from build123d import *
from OCP.BRepAlgoAPI import BRepAlgoAPI_Cut
from OCP.TopTools import TopTools_ListOfShape
from build123d.topology import SkipClean

# Parameters (mm, degrees)
SKETCH1_R                   = 6
EXTRUDE1_DEPTH              = 10
SKETCH2_R                   = 10.75
CUT_EXTRUDE1_DEPTH          = 6
SKETCH3_R                   = 1.6
CUT_EXTRUDE2_DEPTH          = 8.999999347
SKETCH4_W                   = 7
SKETCH4_H                   = 10
SKETCH4_R                   = 1.6
EXTRUDE3_DEPTH              = 9
FILLET2_R                   = 5
CHAMFER4_SIZE               = 6
CHAMFER4_SIZE2              = 10.392304845
M4_TAPPED_HOLE1_D           = 3.3
M4_TAPPED_HOLE1_DEPTH       = 10.1
M4_TAPPED_HOLE1_TIP         = 0.991420021
SKETCH6_R                   = 1.25
EXTRUDE4_DEPTH              = 4
M3_START                    = 12.4999999
M3_TAPPED_HOLE1_OUTLINE_R   = 1.25
M3_TAPPED_HOLE1_DEPTH       = 0.5000001
M3_START_2                  = -13
M3_TAPPED_HOLE1_2_OUTLINE_R = 1.25
M3_TAPPED_HOLE1_2_DEPTH     = 0.4999999
EXTRUDE5_REACH              = 36.756
SKETCH8_W                   = 6
SKETCH8_H                   = 4.052940251


with BuildPart() as part:
    # Sketch1 → Extrude1 (new body)
    with BuildSketch(Plane.XY):
        Polygon((-17, 6.53e-07), (-28, 6.53e-07), (-28, -8.999999347), (28, -8.999999347), (28, 0), (17, 0), (17, 18.000000653), (-17, 18.000000653), align=None)
        with Locations((0, 6.53e-07)):
            Circle(SKETCH1_R, mode=Mode.SUBTRACT)
    extrude(amount=EXTRUDE1_DEPTH)

    # Sketch2 → Cut-Extrude1 (cut)
    with BuildSketch(Plane(origin=(0, 0, 0), x_dir=(-1, 0, 0), z_dir=(0, 0, -1))):
        Circle(SKETCH2_R)
    extrude(amount=-CUT_EXTRUDE1_DEPTH, mode=Mode.SUBTRACT)


with BuildPart() as cut_extrude2_tool:
    # Sketch3 → Cut-Extrude2 (new body)
    with BuildSketch(Plane(origin=(0, 0, 0), x_dir=(-1, 0, 0), z_dir=(0, 1, 0))):
        with Locations(Location((-24.5, 5, 0), (0, 0, 90))):
            Circle(SKETCH3_R)
        with Locations(Location((24.5, 5, 0), (0, 0, 90))):
            Circle(SKETCH3_R)
    extrude(amount=-CUT_EXTRUDE2_DEPTH)


with BuildPart() as part_1:
    add(part.part)

    # Cut-Extrude2: cut by cut_extrude2_tool, with a tolerance
    cut_extrude2_stock = TopTools_ListOfShape()
    cut_extrude2_stock.Append(part_1.part.wrapped)
    cut_extrude2_tools = TopTools_ListOfShape()
    cut_extrude2_tools.Append(cut_extrude2_tool.part.wrapped)
    cut_extrude2_cut = BRepAlgoAPI_Cut()
    cut_extrude2_cut.SetArguments(cut_extrude2_stock)
    cut_extrude2_cut.SetTools(cut_extrude2_tools)
    cut_extrude2_cut.SetFuzzyValue(0.00001)
    cut_extrude2_cut.Build()
    add(Compound.cast(cut_extrude2_cut.Shape()).solids(), mode=Mode.REPLACE)

    # Sketch4 → Extrude3 (add)
    # profile 1 of 2: a face of its own
    with SkipClean():  # the faces are left unmerged after this step: merging them gives an invalid solid
        with BuildSketch(Plane.XZ.offset(8.999999347)):
            with Locations((-24.5, 5)):
                Rectangle(SKETCH4_W, SKETCH4_H)
            with Locations((-24.5, 5)):
                Circle(SKETCH4_R, mode=Mode.SUBTRACT)
        # profile 2 of 2: a face of its own
        with BuildSketch(Plane.XZ.offset(8.999999347)):
            with Locations((24.5, 5)):
                Rectangle(SKETCH4_W, SKETCH4_H)
            with Locations((24.5, 5)):
                Circle(SKETCH4_R, mode=Mode.SUBTRACT)
        extrude(amount=EXTRUDE3_DEPTH)
    add(part_1.part.scale(1), mode=Mode.REPLACE)  # the faces are merged on a copy

    # Fillet2
    fillet2_edges = [part_1.edges().sort_by_distance(p)[0] for p in [
        (28, -13.499999347, 0),
        (28, -13.499999347, 10),
        (-28, -8.999999347, 0),
        (-28, -8.999999347, 10),
    ]]
    fillet(fillet2_edges, radius=FILLET2_R - 0.0001)  # a hair under: the kernel refuses the full size

    # Chamfer4
    chamfer4_edges = [part_1.edges().sort_by_distance(p)[0] for p in [
        (0, 18.000000653, 10),
    ]]
    chamfer4_side = [part_1.faces().sort_by_distance(p)[0] for p in [
        (0, 18.000000653, 5),
    ]]
    chamfer(chamfer4_edges, length=CHAMFER4_SIZE, length2=CHAMFER4_SIZE2, reference=chamfer4_side[0])

    # M4 Tapped Hole1
    with Locations(Plane(origin=(-24.5, -17.999999347, 5), x_dir=(0, 0, -1), z_dir=(0, -1, 0))):
        with Locations((0, 0), (0, 49)):
            Hole(M4_TAPPED_HOLE1_D / 2, depth=M4_TAPPED_HOLE1_DEPTH)
            with Locations((0, 0, -(M4_TAPPED_HOLE1_DEPTH + M4_TAPPED_HOLE1_TIP / 2))):  # 118° drill point
                Cone(0, M4_TAPPED_HOLE1_D / 2, M4_TAPPED_HOLE1_TIP, mode=Mode.SUBTRACT)

    # Sketch6 → Extrude4 (cut)
    with BuildSketch(Plane.ZY.offset(17)):
        with Locations((3.33604719, 14.150000653)):
            Circle(SKETCH6_R)
        with Locations((6.332495088, 8.960000653)):
            Circle(SKETCH6_R)
    extrude4 = extrude(amount=-EXTRUDE4_DEPTH, mode=Mode.SUBTRACT)

    # Mirror1: Extrude4 across plane
    add(extrude4.mirror(Plane(origin=(0, 0, 0), x_dir=(0, 0, 1), z_dir=(1, 0, 0))), mode=Mode.SUBTRACT)

    # M3 Tapped Hole1: read off the stored shape, not the designer's step
    # M3 Tapped Hole1 outline → M3 Tapped Hole1 (cut)
    with SkipClean():  # the faces are left unmerged after this step: merging them gives an invalid solid
        with BuildSketch(Plane.YZ.offset(M3_START)):
            with Locations((14.150000653, 3.33604719)):
                Circle(M3_TAPPED_HOLE1_OUTLINE_R)
            with Locations((8.960000653, 6.332495088)):
                Circle(M3_TAPPED_HOLE1_OUTLINE_R)
        extrude(amount=M3_TAPPED_HOLE1_DEPTH, mode=Mode.SUBTRACT)

    # M3 Tapped Hole1 2 outline → M3 Tapped Hole1 2 (cut)
    with BuildSketch(Plane.YZ.offset(M3_START_2)):
        with Locations((14.150000653, 3.33604719)):
            Circle(M3_TAPPED_HOLE1_2_OUTLINE_R)
        with Locations((8.960000653, 6.332495088)):
            Circle(M3_TAPPED_HOLE1_2_OUTLINE_R)
    extrude(amount=M3_TAPPED_HOLE1_2_DEPTH, mode=Mode.SUBTRACT)

    # M3 Tapped Hole1 3 outline → M3 Tapped Hole1 3 (revolve, cut)
    with BuildSketch(Plane(origin=(0, 14.150000653, 3.33604719), x_dir=(0, 1, 0), z_dir=(0, 0, -1))):
        Polygon((0, 12.5), (0, 11.748924226), (1.25, 12.5), align=None)
        Polygon((1.25, -12.5), (0, -11.748924226), (0, -12.5000001), align=None)
    revolve(axis=Axis((0, 14.150000653, 3.33604719), (1, 0, 0)), mode=Mode.SUBTRACT)

    # M3 Tapped Hole1 4 outline → M3 Tapped Hole1 4 (revolve, cut)
    with BuildSketch(Plane(origin=(0, 8.960000653, 6.332495088), x_dir=(0, 1, 0), z_dir=(0, 0, -1))):
        Polygon((0, 12.5), (0, 11.748924226), (1.25, 12.5), align=None)
        Polygon((1.25, -12.5), (0, -11.748924226), (0, -12.5000001), align=None)
    revolve(axis=Axis((0, 8.960000653, 6.332495088), (1, 0, 0)), mode=Mode.SUBTRACT)

    # Extrude5: up to this plane
    extrude5_end = Plane(origin=(-17, 7.607695808, 10), z_dir=(0, -0.5000000000000007, -0.8660254037844384))
    # Sketch8 → Extrude5 (cut, up to the surface)
    with BuildSketch(Plane(origin=(0, 0, 0), x_dir=(-1, 0, 0), z_dir=(0, 0, -1)), mode=Mode.PRIVATE) as extrude5_sk1:
        with Locations((0, 13.973529875)):
            Rectangle(SKETCH8_W, SKETCH8_H)
    extrude5_tool1 = split(extrude(extrude5_sk1.sketch, amount=-EXTRUDE5_REACH, mode=Mode.PRIVATE), bisect_by=extrude5_end, keep=Keep.BOTH, mode=Mode.PRIVATE)
    add(extrude5_tool1.solids().sort_by_distance((0, 13.97353, 0))[0], mode=Mode.SUBTRACT)


solid = part_1.part
Source: CAD feature listing. Evaluate the final solid. Frame: model axes, mm. A direction names the side the tool comes from. Give positions to 0.01 mm unless a question says otherwise; leave off trailing zeros. Write each loop counter-clockwise with the first axis right and the second up, starting at its lowest first coordinate (ties: lowest second). Pieces come first, ordered by that corner, then holes. Notation, with made-up numbers: M -39.75,34 L -18.75,34 A29 ccw -18.75,73 Z; hole C 35,70.5 d10. An arc over 180 degrees is marked long. Answer as a JSON object with one key per item and string values.
Q1. Mould query, pull axis X, two halves, no side actions, for faces 5 (the face through (11.88, 8.8, 6.48)), 6 (the face through (-27, -9, 2)), 7 (the face through (0, 16, 3)). Classes: +X half, -X half, draft (parallel to the pull), parting line (faces both ways), or undercut.
Geometry check:
{"face 5": "+X half", "face 6": "-X half", "face 7": "undercut"}
Q2. Cut plane B-B, the plane x = 0. Return the cut outline in (y, z), then the cut area to 3 significant figures.
Geometry check:
{"outline": "M -9,6 L -6,6 L -6,10 L -9,10 Z; M 6,6 L 10.75,6 L 10.75,0 L 11.95,0 L 11.95,7.49 L 7.61,10 L 6,10 Z; M 16,0 L 18,0 L 18,4 L 16,5.15 Z", "area": "46.7 mm^2"}
Q3. Cut plane D-D, the plane z = 8.5. Return the cut outline in (x, y), then the cut area to 3 significant figures.
Geometry check:
{"outline": "M -26.57,-18 L -21,-18 L -21,-9 L 21,-9 L 21,-18 L 26.57,-18 L 26.57,0 L 17,0 L 17,10.21 L -17,10.21 L -17,0 L -26.57,0 Z; hole C 0,0 d12", "area": "812 mm^2"}
Q4. Ray query, line 1 along X through (y, z) = (-15.25, 5); line 2 along X through (y, z) = (-5, 5); line 3 along Y through (x, z) = (-13.5, 1). Return the intervals inside material, ascending.
Geometry check:
{"line 1": "x = -28 to -26.15, -22.85 to -21, 21 to 22.85, 26.15 to 28", "line 2": "x = -28 to -26.1, -22.9 to -9.52, 9.52 to 22.9, 26.1 to 28", "line 3": "y = -9 to 18"}
Q5. Access query for faces 1 (the face through (3, -6, 6)), 2 (the face through (-22, 0, 5)), 3 (the face through (21, -13, 5)), 4 (the face through (3, 14, 3)). Directions: +Z, -Z, +X, -X, +Y, -Y. A direction counts if a zero-diameter tool reaches every point of the face in a straight line with its end or side. Return the directions, or none.
Geometry check:
{"face 1": "-Z", "face 2": "+Z, -Z, -X, +Y", "face 3": "+Z, -Z, -Y", "face 4": "+Z, -Z"}
Q6. Cut plane A-A, the plane y = -12.5. Count the separate pieces of the cut face and the enclosed holes in it, then the cut area to 3 significant figures.
Geometry check:
{"separate pieces": "2", "enclosed holes": "2", "area": "101 mm^2"}
Q7. Contact query for flat-ended pins moving along their axis: P1, Ø2, axis at y = 14.15, z = 3.34, coming from the -X side; P2, Ø2, axis at x = 19, z = 6.5, coming from the -Y side; P3, Ø3, axis at y = 8.96, z = 6.33, coming from the +X side. Output: stop coordinate, or through.
Geometry check:
{"P1": "stops at x = -12.35", "P2": "stops at y = -9", "P3": "stops at x = 17"}
